Here's how the part is built. I have some questions about the finished solid (model axes, mm). Face numbers are marked on the shaded views. A direction names the side the tool comes from. Round coordinates to 2 decimals unless told otherwise and drop trailing zeros. Write each loop counter-clockwise with the first axis right and the second up, starting at its lowest first coordinate (ties: lowest second). Pieces come first, ordered by that corner, then holes. Notation, with made-up numbers: (40.5, 71.25) -> (77.5, 71.25) arc R16 cw to (77.5, 95.25) -> close; hole circle Ø3 at (4.25, 75.25). An arc over 180 degrees is marked (long way). Put each result on its own line as item: value. Start each with the question number.
1. Which directions (+Z, -Z, +X, -X, +Y, -Y) give clear straight access to the entire face, cutting with the end or side of a thin tool? Please do the marked faces 4 and 5.
2. Suppose I cut it at B-B (z = 0). Please give me the cut outline in (x, y).
3. We'd pull the mould along X, two halves only. Please class the marked faces 1, 2 and 3: +X half, -X half, draft (parallel to the pull), parting line (faces both ways), or undercut.
4. I need wall thicknesses on probe 1 along X at (y, z) = (4.3, 11.25); probe 2 along X at (y, z) = (2.5, -10); probe 3 along Y at (x, z) = (5, 11.5). Which ranges of each line are inside material? Lowest first, please. Write a range as from..to.
5. For pin 1 (10 mm diameter, centred on x = -11.5, y = 19, fed in from -Z); pin 2 (6 mm diameter, centred on x = 19.49, z = -11.25, fed in from +Y); pin 3 (1 mm diameter, centred on x = 11, y = 8, fed in from +Z), each with a flat end and sliding along its axis, tell me the tip position at first contact or that it passes through.
6. Suppose I cut it at D-D (x = 9.5). Please give me the cut outline in (y, z), then the cut area to 3 significant figures.
7. Suppose I cut it at A-A (x = 0). Please give me the cut outline in (y, z), then the cut area to 3 significant figures.
8. Suppose I cut it at C-C (y = 2.5). Please give me the cut outline in (x, z).
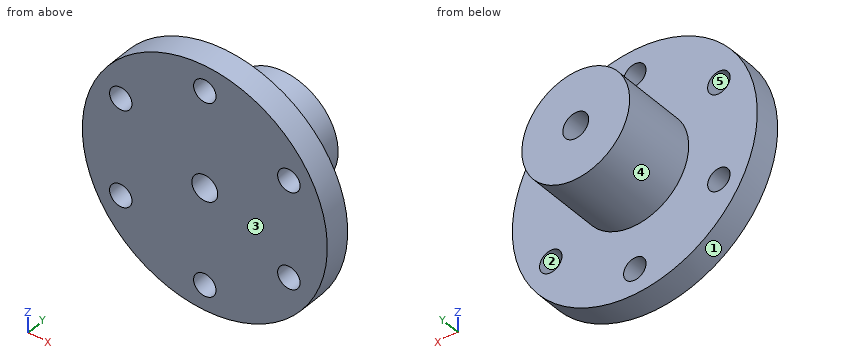
```python
from build123d import *

# Parameters (mm, degrees)
SKETCH_1_R          = 28.4
EXTRUDE_1_DEPTH     = 6
SKETCH_2_R          = 12.5
EXTRUDE_2_DEPTH     = 17.4
SKETCH_3_R          = 3
CUT_EXTRUDE_1_DEPTH = 60
SKETCH_4_R          = 2.6
CUT_EXTRUDE_2_DEPTH = 10


with BuildPart() as part:
    # 草图1 → 凸台-拉伸1 (new body)
    with BuildSketch(Plane(origin=(0, 0, 0), x_dir=(1, 0, 0), z_dir=(0, 1, 0))):
        with Locations(Location((0, 0, 0), (0, 0, 270))):
            Circle(SKETCH_1_R)
    extrude(amount=EXTRUDE_1_DEPTH)

    # 草图2 → 凸台-拉伸2 (add)
    with BuildSketch(Plane(origin=(0, 6, 0), x_dir=(1, 0, 0), z_dir=(0, 1, 0))):
        with Locations(Location((0, 0, 0), (0, 0, 270))):
            Circle(SKETCH_2_R)
    extrude(amount=EXTRUDE_2_DEPTH)

    # 草图3 → 切除-拉伸1 (cut)
    with BuildSketch(Plane(origin=(0, 23.4, 0), x_dir=(1, 0, 0), z_dir=(0, 1, 0))):
        with Locations(Location((0, 0, 0), (0, 0, 270))):
            Circle(SKETCH_3_R)
    extrude(amount=-CUT_EXTRUDE_1_DEPTH, mode=Mode.SUBTRACT)

    # 草图4 → 切除-拉伸2 (cut)
    with BuildSketch(Plane.XZ):
        with Locations(Location((0, 22.5, 0), (0, 0, 270))):
            Circle(SKETCH_4_R)
        with Locations(Location((19.485571585, 11.25, 0), (0, 0, 270))):
            Circle(SKETCH_4_R)
        with Locations(Location((19.485571585, -11.25, 0), (0, 0, 270))):
            Circle(SKETCH_4_R)
        with Locations(Location((0, -22.5, 0), (0, 0, 270))):
            Circle(SKETCH_4_R)
        with Locations(Location((-19.485571585, -11.25, 0), (0, 0, 270))):
            Circle(SKETCH_4_R)
        with Locations(Location((-19.485571585, 11.25, 0), (0, 0, 270))):
            Circle(SKETCH_4_R)
    extrude(amount=-CUT_EXTRUDE_2_DEPTH, mode=Mode.SUBTRACT)


solid = part.part
```
Verdict:
1. face 4: +Y
1. face 5: +Y, -Y
2. outline: (-28.4, 0) -> (-3, 0) -> (-3, 23.4) -> (-12.5, 23.4) -> (-12.5, 6) -> (-28.4, 6) -> close; (3, 0) -> (28.4, 0) -> (28.4, 6) -> (12.5, 6) -> (12.5, 23.4) -> (3, 23.4) -> close
3. face 1: parting line
3. face 2: undercut
3. face 3: draft
4. probe 1: x = -26.08..-22.09, -16.89..16.89, 22.09..26.08
4. probe 2: x = -26.58..-21.77, -17.21..17.21, 21.77..26.58
4. probe 3: y = 0..6
5. pin 1: stops at z = -10.68
5. pin 2: stops at y = 6
5. pin 3: stops at z = 6.78
6. outline: (0, -26.76) -> (6, -26.76) -> (6, -8.12) -> (23.4, -8.12) -> (23.4, 8.12) -> (6, 8.12) -> (6, 26.76) -> (0, 26.76) -> close
6. area: 604 mm^2
7. outline: (0, -28.4) -> (6, -28.4) -> (6, -25.1) -> (0, -25.1) -> close; (0, -19.9) -> (6, -19.9) -> (6, -12.5) -> (23.4, -12.5) -> (23.4, -3) -> (0, -3) -> close; (0, 3) -> (23.4, 3) -> (23.4, 12.5) -> (6, 12.5) -> (6, 19.9) -> (0, 19.9) -> close; (0, 25.1) -> (6, 25.1) -> (6, 28.4) -> (0, 28.4) -> close
7. area: 573 mm^2
8. outline: circle Ø56.8 at (0, 0); hole circle Ø5.2 at (-19.49, -11.25); hole circle Ø5.2 at (-19.49, 11.25); hole circle Ø6 at (0, 0); hole circle Ø5.2 at (0, -22.5); hole circle Ø5.2 at (0, 22.5); hole circle Ø5.2 at (19.49, -11.25); hole circle Ø5.2 at (19.49, 11.25)
